Verification items for the finished model (mm, model axes). A direction names the side the tool comes from. Give positions to 0.01 mm unless a question says otherwise; leave off trailing zeros. Loops run counter-clockwise (first coordinate to the right, second up) from the corner with the lowest first, then second, coordinate; pieces in that order, holes last. Notation, with made-up numbers: M 59.25,50.25 L 83.25,50.25 A16 cw 83.25,77.25 Z; hole C 64,49 d5. An arc over 180 degrees is marked long. Answer in a Markdown table with one row per item.
```python
from build123d import *

# Parameters (mm, degrees)
BOSS_EXTRUDE1_DEPTH = 2
BOSS_EXTRUDE2_DEPTH = 2.54
SKETCH3_R           = 3.175
BOSS_EXTRUDE3_DEPTH = 6.35


with BuildPart() as part:
    # Sketch1 → Boss-Extrude1 (new body)
    with BuildSketch(Plane.XY):
        with BuildLine():
            Line((6.058373601, -6.598394326), (21.020213328, -4.31191015))
            ThreePointArc((21.020213328, -4.31191015), (24.724999848, 0.002643865), (21.019053909, 4.316202049))
            Line((21.019053909, 4.316202049), (6.056600222, 6.598665092))
            ThreePointArc((6.056600222, 6.598665092), (5.05, 6.675), (4.043399778, 6.598665092))
            Line((4.043399778, 6.598665092), (-10.919053909, 4.316202049))
            ThreePointArc((-10.919053909, 4.316202049), (-14.624999848, 0.002643865), (-10.920213328, -4.31191015))
            Line((-10.920213328, -4.31191015), (4.041626399, -6.598394326))
            ThreePointArc((4.041626399, -6.598394326), (5.05, -6.675), (6.058373601, -6.598394326))
        make_face()
        with BuildLine():
            Line((20.63601802, 1.80524934), (5.673564332, 4.087712383))
            ThreePointArc((5.673564332, 4.087712383), (5.05, 4.135), (4.426435668, 4.087712383))
            Line((4.426435668, 4.087712383), (-10.53601802, 1.80524934))
            ThreePointArc((-10.53601802, 1.80524934), (-12.084999871, 0.002302548), (-10.536502624, -1.801060474))
            Line((-10.536502624, -1.801060474), (4.425337102, -4.08754465))
            ThreePointArc((4.425337102, -4.08754465), (5.05, -4.135), (5.674662898, -4.08754465))
            Line((5.674662898, -4.08754465), (20.636502624, -1.801060474))
            ThreePointArc((20.636502624, -1.801060474), (22.184999871, 0.002302548), (20.63601802, 1.80524934))
        make_face(mode=Mode.SUBTRACT)
    extrude(amount=BOSS_EXTRUDE1_DEPTH)

    # Sketch2 → Boss-Extrude2 (add)
    with BuildSketch(Plane.XY.offset(2)):
        with BuildLine():
            Line((6.058373601, -6.598394326), (21.020213328, -4.31191015))
            ThreePointArc((21.020213328, -4.31191015), (24.724999848, 0.002643865), (21.019053909, 4.316202049))
            Line((21.019053909, 4.316202049), (6.056600222, 6.598665092))
            ThreePointArc((6.056600222, 6.598665092), (5.05, 6.675), (4.043399778, 6.598665092))
            Line((4.043399778, 6.598665092), (-10.919053909, 4.316202049))
            ThreePointArc((-10.919053909, 4.316202049), (-14.624999848, 0.002643865), (-10.920213328, -4.31191015))
            Line((-10.920213328, -4.31191015), (4.041626399, -6.598394326))
            ThreePointArc((4.041626399, -6.598394326), (5.05, -6.675), (6.058373601, -6.598394326))
        make_face()
    extrude(amount=BOSS_EXTRUDE2_DEPTH)

    # Sketch3 → Boss-Extrude3 (add)
    with BuildSketch(Plane.XY.offset(4.54)):
        with Locations((19.761311468, 0)):
            Circle(SKETCH3_R)
    extrude(amount=BOSS_EXTRUDE3_DEPTH)


solid = part.part
```
Item 1: Release check for a two-part mould opening along Y. For faces 4 (the cylindrical face through (5.036, -6.675, 2.238)), 5 (the cylindrical face through (5.059, 4.135, 0.986)), 6 (the flat face through (-3.333, 5.473, 2.238)) record: released by +Y, released by -Y, zero draft, split by the parting line, or undercut.
Reported:
| item | result |
|---|---|
| face 4 | released by -Y |
| face 5 | undercut |
| face 6 | released by +Y |
Item 2: Tool access check on faces 1 (the flat face through (20, 0, 10.89)), 2 (the cylindrical face through (22.7, -1.2, 7.7)), 3 (the flat face through (13.26, 2.93, 0.99)). Record the directions out of +Z, -Z, +X, -X, +Y, -Y that give a thin tool (end or side, any length) a straight path to the whole face; none if there is none.
Reported:
| item | result |
|---|---|
| face 1 | +Z, +X, -X, +Y, -Y |
| face 2 | +Z |
| face 3 | -Z |
Item 3: Sectioned sample at D-D (y = -2.25). Record the cut outline in (x, z), and give its area (3 significant figures).
Reported:
| item | result |
|---|---|
| outline | M -14,0 L -7.6,0 L -7.6,2 L 17.7,2 L 17.7,0 L 24.1,0 L 24.1,4.54 L 22,4.54 L 22,10.89 L 17.52,10.89 L 17.52,4.54 L -14,4.54 Z |
| area | 151 mm^2 |
Item 4: Sectioned sample at C-C (x = -5). Record the cut outline in (y, z), and give its area (3 significant figures).
Reported:
| item | result |
|---|---|
| outline | M -5.22,0 L -2.65,0 L -2.65,2 L 2.65,2 L 2.65,0 L 5.22,0 L 5.22,4.54 L -5.22,4.54 Z |
| area | 36.8 mm^2 |
Item 5: Go/stop test with flat-tipped pins: pin 1 (3 mm diameter, centred on y = 2.5, z = 8.5, fed in from +X); pin 2 (6 mm diameter, centred on x = 13, y = -4, fed in from +Z); pin 3 (5 mm diameter, centred on x = -1.5, z = 1.5, fed in from +Y). Record where each tip stops, or that it passes through.
Reported:
| item | result |
|---|---|
| pin 1 | stops at x = 22.77 |
| pin 2 | stops at z = 4.54 |
| pin 3 | stops at y = 6.13 |
Item 6: Scan lines: L1, parallel to Y at x = -4, z = 0.5; L2, parallel to Z at x = 4, y = 0; L3, parallel to Z at x = 15.5, y = 3. Record each from-to range of solid material in increasing order. Write a range as [from, to].
Reported:
| item | result |
|---|---|
| L1 | y = [-5.37, -2.8], [2.8, 5.37] |
| L2 | z = [2, 4.54] |
| L3 | z = [0, 4.54] |
Item 7: Sectioned sample at B-B (y = 0). Record the cut outline in (x, z) (3 decimals).
Reported:
| item | result |
|---|---|
| outline | M -14.625,0 L -12.085,0 L -12.085,2 L 22.185,2 L 22.185,0 L 24.725,0 L 24.725,4.54 L 22.936,4.54 L 22.936,10.89 L 16.586,10.89 L 16.586,4.54 L -14.625,4.54 Z |
Item 8: Sectioned sample at A-A (z = 2.75). Record the cut outline in (x, y) (3 decimals), and give its area (3 significant figures).
Reported:
| item | result |
|---|---|
| outline | M -10.92,-4.312 L 4.042,-6.598 A6.675 ccw 6.058,-6.598 L 21.02,-4.312 A4.364 ccw 21.019,4.316 L 6.057,6.599 A6.675 ccw 4.043,6.599 L -10.919,4.316 A4.364 ccw Z |
| area | 402 mm^2 |
